Here's how the part is built. I have some questions about the finished solid (model axes, mm). A direction names the side the tool comes from. Give positions to 0.01 mm unless a question says otherwise; leave off trailing zeros. Write each loop counter-clockwise with the first axis right and the second up, starting at its lowest first coordinate (ties: lowest second). Pieces come first, ordered by that corner, then holes. Notation, with made-up numbers: (-19.75, 72) - (-1.75, 72) arc R31 cw to (-1.75, 108) - close; hole circle Ø7 at (80.5, 5.25). An arc over 180 degrees is marked (long way). Use one line per item in the form item = value. Start each with the question number.
from build123d import *

# Parameters (mm, degrees)
BOSS_EXTRUDE1_DEPTH   = 2
BOSS_EXTRUDE1_2_DEPTH = 2
BOSS_EXTRUDE2_DEPTH   = 10
SKETCH1_4_R           = 16
BOSS_EXTRUDE3_DEPTH   = 2


with BuildPart() as part:
    # Sketch1 → Boss-Extrude1 (new body)
    with BuildSketch(Plane(origin=(0, 0, 0), x_dir=(0, 1, 0), z_dir=(0, 0, 1))):
        with BuildLine():
            ThreePointArc((13.678815738, -11.7), (0, -18), (-13.678815738, -11.7))
            Line((-13.678815738, -11.7), (-3.799671038, -23.25))
            ThreePointArc((-3.799671038, -23.25), (0, -25), (3.799671038, -23.25))
            Line((3.799671038, -23.25), (13.678815738, -11.7))
        make_face()
    extrude(amount=-BOSS_EXTRUDE1_DEPTH)



with BuildPart() as body_2:
    # Sketch1 → Boss-Extrude1 2 (new body)
    with BuildSketch(Plane(origin=(0, 0, 0), x_dir=(0, 1, 0), z_dir=(0, 0, 1))):
        with BuildLine():
            ThreePointArc((3.799671038, 23.25), (0, 25), (-3.799671038, 23.25))
            Line((-3.799671038, 23.25), (-13.678815738, 11.7))
            ThreePointArc((-13.678815738, 11.7), (0, 18), (13.678815738, 11.7))
            Line((13.678815738, 11.7), (3.799671038, 23.25))
        make_face()
    extrude(amount=-BOSS_EXTRUDE1_2_DEPTH)


with BuildPart() as part_1:
    add(part.part)

    add(body_2.part)  # Boss-Extrude2 merges body 2
    # Sketch1_3 → Boss-Extrude2 (add)
    with BuildSketch(Plane(origin=(0, 0, 0), x_dir=(0, 1, 0), z_dir=(0, 0, 1))):
        with BuildLine():
            ThreePointArc((-16, 0), (0, 16), (16, 0))
            Line((16, 0), (18, 0))
            ThreePointArc((18, 0), (16.885181126, 6.236237516), (13.678815738, 11.7))
            ThreePointArc((13.678815738, 11.7), (0, 18), (-13.678815738, 11.7))
            ThreePointArc((-13.678815738, 11.7), (-16.885181126, 6.236237516), (-18, 0))
            Line((-18, 0), (-16, 0))
        make_face()
        with BuildLine():
            Line((18, 0), (16, 0))
            ThreePointArc((16, 0), (0, -16), (-16, 0))
            Line((-16, 0), (-18, 0))
            ThreePointArc((-18, 0), (-16.885181126, -6.236237516), (-13.678815738, -11.7))
            ThreePointArc((-13.678815738, -11.7), (0, -18), (13.678815738, -11.7))
            ThreePointArc((13.678815738, -11.7), (16.885181126, -6.236237516), (18, 0))
        make_face()
    extrude(amount=-BOSS_EXTRUDE2_DEPTH)

    # Sketch1_4 → Boss-Extrude3 (add)
    with BuildSketch(Plane(origin=(0, 0, 0), x_dir=(0, 1, 0), z_dir=(0, 0, 1))):
        with Locations(Location((0, 0, 0), (0, 0, 270))):
            Circle(SKETCH1_4_R)
    extrude(amount=-BOSS_EXTRUDE3_DEPTH)


solid = part_1.part
1. I want a section at B-B, the plane z = -4.5. List the corners of the cut face in (x, y) for me, then the cut area to 3 significant figures.
2. For faces 5 (the face through (6.13, -14.78, -5.94)), 6 (the face through (11, -12, -10)), 7 (the face through (-20, 0, -2)), which set-ups out of +Z, -Z, +X, -X, +Y, -Y let a thin tool reach every point of the face, with its end or its side?
3. For P1, Ø2, axis at x = -11, y = -1, coming from the +Z side; P2, Ø1.5, axis at y = -4, z = -8, coming from the +X side; P3, Ø9.5, axis at x = 7, y = -3.5, coming from the -Z side; P4, Ø2, axis at y = 3, z = -4.5, coming from the -X side, each with a flat end and sliding along its axis, tell me the tip position at first contact or that it passes through.
4. I want a section at A-A, the plane y = 0. List the corners of the cut face in (x, z) for me, then the cut area to 3 significant figures.
5. I want a section at C-C, the plane z = -1. List the corners of the cut face in (x, y) for me, then the cut area to 3 significant figures.
6. Please list where these lines run through material, in increasing order: line 1 (X direction, y = 0, z = -7); line 2 (Z direction, x = -4, y = 13.5); line 3 (Y direction, x = 1, z = -3.25).
7. I want a section at D-D, the plane x = -11. List the corners of the cut face in (y, z) for me.
8. We'd pull the mould along Y, two halves only. Please class faces 1 (the face through (25, 0, -1)), 2 (the face through (0, 0, -2)), 3 (the face through (0, 0, 0)), 4 (the face through (-17.556, -8.67, -0.986)): pulls with the +Y half, pulls with the -Y half, needs draft (parallel to the pull), parting line crosses it, or undercut.
Result sheet:
q1.outline = circle Ø36 at (0, 0); hole circle Ø32 at (0, 0)
q1.area = 214 mm2
q2.face_5 = -Z
q2.face_6 = -Z, +X, -X, +Y, -Y
q2.face_7 = -Z, -X
q3.P1 = 0
q3.P2 = 17.7
q3.P3 = -2
q3.P4 = -17.89
q4.outline = (-25, -2) - (-18, -2) - (-18, -10) - (-16, -10) - (-16, -2) - (16, -2) - (16, -10) - (18, -10) - (18, -2) - (25, -2) - (25, 0) - (-25, 0) - close
q4.area = 132 mm2
q5.outline = (-23.25, -3.8) - (-11.7, -13.68) arc R18 ccw to (11.7, -13.68) - (23.25, -3.8) arc R5 ccw to (23.25, 3.8) - (11.7, 13.68) arc R18 ccw to (-11.7, 13.68) - (-23.25, 3.8) arc R5 ccw to start
q5.area = 1,200 mm2
q6.line_1 = -18 to -16, 16 to 18
q6.line_2 = -2 to 0
q6.line_3 = -17.97 to -15.97, 15.97 to 17.97
q7.outline = (-14.25, -10) - (-11.62, -10) - (-11.62, -2) - (11.62, -2) - (11.62, -10) - (14.25, -10) - (14.25, 0) - (-14.25, 0) - close
q8.face_1 = parting line crosses it
q8.face_2 = undercut
q8.face_3 = needs draft
q8.face_4 = pulls with the -Y half
